Geometry check sheet. Reference: drawing and pictorial views, mm from the part's lowest x, y, z. Coordinates: 2 decimals unless noted, no trailing zeros. Loops run counter-clockwise (first coordinate to the right, second up) from the corner with the lowest first, then second, coordinate; pieces in that order, holes last. Notation, with made-up numbers: (-32.5, -31) -> (15.5, -31) arc R10 cw to (15.5, -16) -> close; hole circle Ø1 at (-21.5, 10). An arc over 180 degrees is marked (long way). Answer as a JSON object with one key per item and string values.
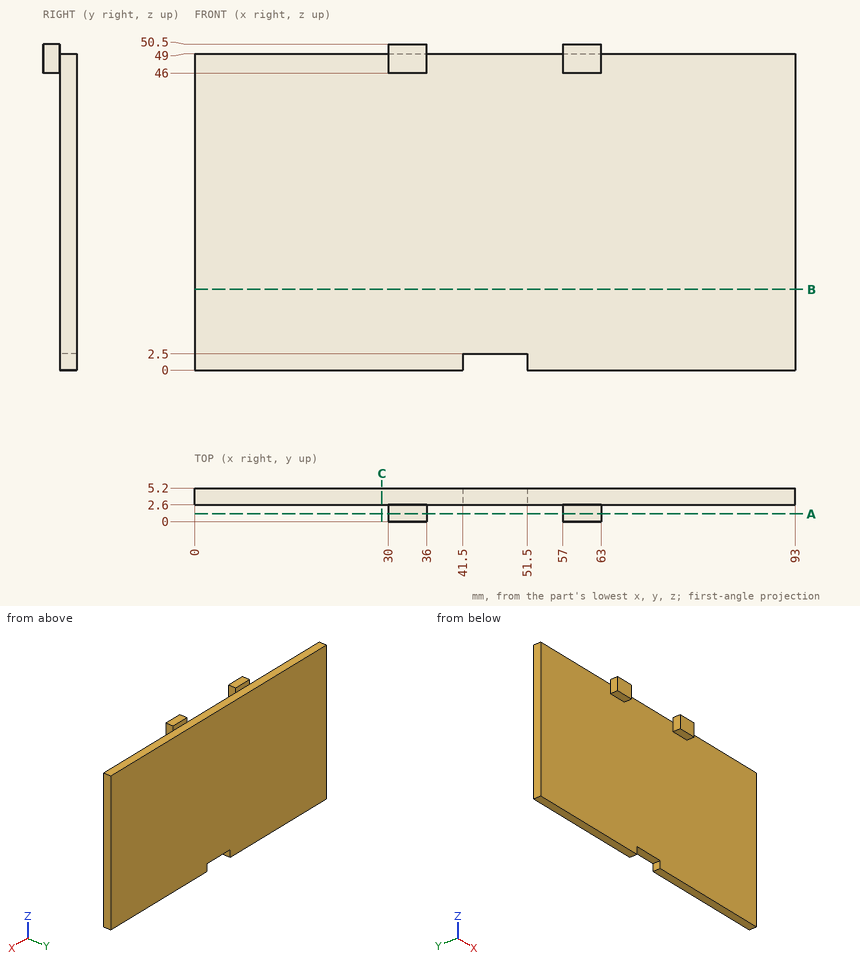
1. Section check C-C, the plane x = 29. Record the boundary of the cut face in (y, z), then the cut area to 3 significant figures.
Evaluation:
{"outline": "(2.6, 0) -> (5.2, 0) -> (5.2, 49) -> (2.6, 49) -> close", "area": "127 mm^2"}
2. Section check B-B, the plane z = 12.5. Record the boundary of the cut face in (x, y).
Evaluation:
{"outline": "(0, 2.6) -> (93, 2.6) -> (93, 5.2) -> (0, 5.2) -> close"}
3. Depth check by flat-ended pin: P1, Ø0.8, axis at x = 59.5, z = 50, coming from the +Y side; P2, Ø1.3, axis at y = 0.5, z = 48, coming from the -X side; P3, Ø0.8, axis at y = 1, z = 47.5, coming from the +X side; P4, Ø3, axis at y = 1, z = 13.5, coming from the -X side. Enter the tip coordinate at first touch or a pass-through.
Evaluation:
{"P1": "stops at y = 2.6", "P2": "stops at x = 30", "P3": "stops at x = 63", "P4": "passes through"}
4. Thickness scan on probe 1 along X at (y, z) = (1.6, 47); probe 2 along Y at (x, z) = (6, 19); probe 3 along Z at (x, y) = (18.5, 4.4). Record the ranges inside material, lowest first. Write a range as from..to.
Evaluation:
{"probe 1": "x = 30..36, 57..63", "probe 2": "y = 2.6..5.2", "probe 3": "z = 0..49"}
5. Section check A-A, the plane y = 1.2. Record the boundary of the cut face in (x, z), then the cut area to 3 significant figures.
Evaluation:
{"outline": "(30, 46) -> (36, 46) -> (36, 50.5) -> (30, 50.5) -> close; (57, 46) -> (63, 46) -> (63, 50.5) -> (57, 50.5) -> close", "area": "54.0 mm^2"}
